Input: dimensioned drawing with shaded views. Units: mm. Origin: part minimum x, y, z. Give positions to 0.01 mm unless a question says otherwise; leave off trailing zeros. Loops run counter-clockwise (first coordinate to the right, second up) from the corner with the lowest first, then second, coordinate; pieces in that order, holes last. Notation, with made-up numbers: (84.25, -39) -> (112.25, -39) arc R28 cw to (112.25, -15) -> close; hole circle Ø7 at (87, 72.25). An arc over 180 degrees is marked (long way). Answer in a Markdown table with one row per item. Add a question column.
1) Section query B-B (y = 9.25). Return the cut outline in (x, z) (1 decimal).
2) Draft query along X for the marked faces 1, 2, 3 and 4. Return one class per face: +X half, -X half, draft (parallel to the pull), parting line (faces both ways), or undercut.
3) Section query C-C (y = 5.25). Return the cut outline in (x, z) (1 decimal), plus the area to 3 significant figures.
4) Section query D-D (z = 0.9). Give the number of separate pieces and of enclosed holes in the cut face, plus the area to 3 significant figures.
5) Section query A-A (x = 24.13). Return the cut outline in (y, z) (1 decimal).
6) First-contact query: P1, Ø1.9, axis at x = 24.13, y = 6.35, coming from the -Z side. Flat tip, straight axial feed; report the tip coordinate or a pass-through.
7) Line query: line 1 (X direction, y = 9.5, z = 0.4); line 2 (X direction, y = 6, z = 1.5) (1 decimal); line 3 (Y direction, x = 13.75, z = 0.25) (1 decimal). Output: solid intervals per line, ascending. Write a range as from..to.
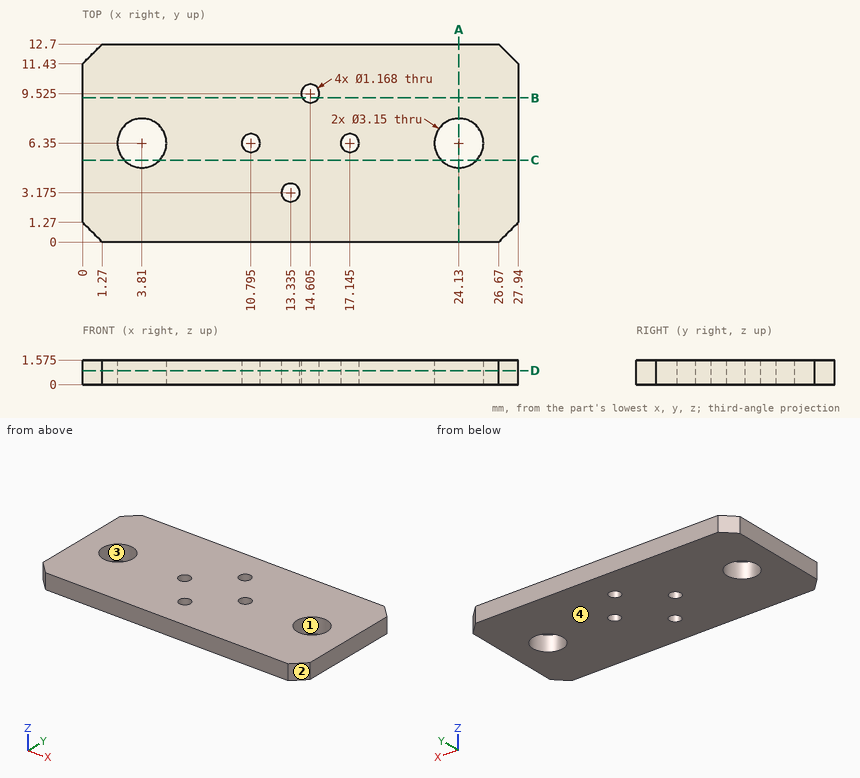
Evaluation:
| question | item | result |
|---|---|---|
| 1 | outline | (0, 0) -> (14.1, 0) -> (14.1, 1.6) -> (0, 1.6) -> close; (15.1, 0) -> (27.9, 0) -> (27.9, 1.6) -> (15.1, 1.6) -> close |
| 2 | face 1 | undercut |
| 2 | face 2 | +X half |
| 2 | face 3 | undercut |
| 2 | face 4 | draft |
| 3 | outline | (0, 0) -> (2.7, 0) -> (2.7, 1.6) -> (0, 1.6) -> close; (4.9, 0) -> (23, 0) -> (23, 1.6) -> (4.9, 1.6) -> close; (25.3, 0) -> (27.9, 0) -> (27.9, 1.6) -> (25.3, 1.6) -> close |
| 3 | area | 36.9 mm² |
| 4 | separate pieces | 1 |
| 4 | enclosed holes | 6 |
| 4 | area | 332 mm² |
| 5 | outline | (0, 0) -> (4.8, 0) -> (4.8, 1.6) -> (0, 1.6) -> close; (7.9, 0) -> (12.7, 0) -> (12.7, 1.6) -> (7.9, 1.6) -> close |
| 6 | P1 | through |
| 7 | line 1 | 0..14.02, 15.19..27.94 |
| 7 | line 2 | 0..2.3, 5.3..10.3, 11.3..16.7, 17.6..22.6, 25.7..27.9 |
| 7 | line 3 | 0..2.8, 3.6..12.7 |
